from build123d import *

# Parameters (mm, degrees)
F0_R     = 17.5
F1_DEPTH = 60
F3_DEPTH = 11.8
F4_R     = 2.85
F5_DEPTH = 6
F6_SIZE  = 1
F7_SIZE  = 0.5
F8_SIZE  = 2


with BuildPart() as f1:
    # F0 (on Top) → F1 (new body)
    with BuildSketch(Plane.XY):
        Circle(F0_R)
    extrude(amount=F1_DEPTH)

    # F2 (on face) → F3 (join)
    with BuildSketch(Plane.XY.offset(60)):
        with BuildLine():
            ThreePointArc((-2.3867830802, 11.1984716157), (-7.2032573788, -8.9003136537), (11.45, 0))
            ThreePointArc((11.45, 0), (8.9003136537, 7.2032573788), (2.3867830802, 11.1984716157))
            ThreePointArc((2.3867830802, 11.1984716157), (0, 9.05), (-2.3867830802, 11.1984716157))
        make_face()
        with BuildLine():
            ThreePointArc((-2.3867830802, 11.1984716157), (0, 9.05), (2.3867830802, 11.1984716157))
            ThreePointArc((2.3867830802, 11.1984716157), (0, 11.45), (-2.3867830802, 11.1984716157))
        make_face()
        with BuildLine():
            ThreePointArc((-2.3867830802, 11.1984716157), (0, 11.45), (2.3867830802, 11.1984716157))
            ThreePointArc((2.3867830802, 11.1984716157), (2.3966934923, 11.324062302), (2.4, 11.45))
            ThreePointArc((2.4, 11.45), (-0.125937698, 13.8466934923), (-2.3867830802, 11.1984716157))
        make_face()
    extrude(amount=F3_DEPTH)

    # F4 (on face) → F5 (join)
    with BuildSketch(Plane.XY.offset(71.8)):
        Circle(F4_R)
    extrude(amount=F5_DEPTH)

    # F6
    f6_edges = [f1.edges().sort_by_distance(p)[0] for p in [
        (-2.85, 0, 77.8),
    ]]
    chamfer(f6_edges, length=F6_SIZE)

    # F7
    f7_edges = [f1.edges().sort_by_distance(p)[0] for p in [
        (0, -11.45, 71.8),
        (0, 13.85, 71.8),
        (-17.5, 0, 60),
    ]]
    chamfer(f7_edges, length=F7_SIZE)

    # F8
    f8_edges = [f1.edges().sort_by_distance(p)[0] for p in [
        (-17.5, 0, 0),
    ]]
    chamfer(f8_edges, length=F8_SIZE)


solid = f1.part
Design review of the part built by this model. Coordinates are the model's own, in mm. A direction names the side the tool comes from. Coordinates: 2 decimals unless noted, no trailing zeros. Loops run counter-clockwise (first coordinate to the right, second up) from the corner with the lowest first, then second, coordinate; pieces in that order, holes last.
Item 1: Add section B-B (z = 45.5). Write out the cut boundary in (x, y).
Completed:
outline: circle Ø35 at (0, 0)
Item 2: Wall thickness on L1, parallel to Z at x = -2, y = -10.5; L2, parallel to Z at x = -11, y = -5.5; L3, parallel to Y at x = 0.5, z = 36.5: over which ranges is each line inside the solid? List them lowest first.
Completed:
L1: z = 0 to 71.8
L2: z = 0 to 60
L3: y = -17.49 to 17.49
Item 3: For faces 1 (the cylindrical face through (-13.887, -10.648, 30.348)), 2 (the flat face through (4, -11, 60)), list the 3-axis set-ups (+Z, -Z, +X, -X, +Y, -Y) from which the entire face can be reached by the end or side of a thin tool; tool diameter is ignored.
Completed:
face 1: +Z, -Z
face 2: +Z
Item 4: Add section A-A (x = 0). Write out the cut boundary in (y, z), and give its area (3 significant figures).
Completed:
outline: (-17.5, 2) - (-15.5, 0) - (15.5, 0) - (17.5, 2) - (17.5, 59.5) - (17, 60) - (13.85, 60) - (13.85, 71.3) - (13.35, 71.8) - (2.85, 71.8) - (2.85, 76.8) - (1.85, 77.8) - (-1.85, 77.8) - (-2.85, 76.8) - (-2.85, 71.8) - (-10.95, 71.8) - (-11.45, 71.3) - (-11.45, 60) - (-17, 60) - (-17.5, 59.5) - close
area: 2,430 mm2
Item 5: Clearance check with flat-ended pins moving along their axes: pin 1 (1.5 mm diameter, centred on x = -7.5, y = 0, fed in from +Z); pin 2 (1 mm diameter, centred on y = 1, z = 67.5, fed in from +X); pin 3 (5 mm diameter, centred on x = -13.5, y = 13, fed in from +Z). State where each tip first meets the part, or that it passes through.
Completed:
pin 1: stops at z = 71.8
pin 2: stops at x = 11.44
pin 3: stops at z = 60
